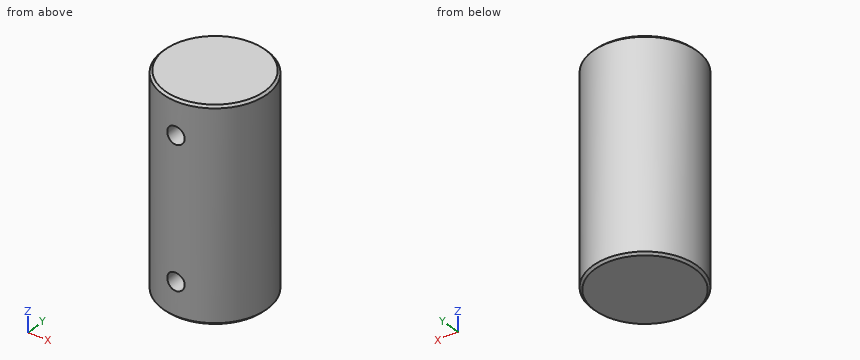
```python
from build123d import *

# Parameters (mm, degrees)
SKETCH1_R         = 9.525
EXTRUDE1_DEPTH    = 19.05
CHAMFER1_SIZE     = 0.4064
SKETCH6_R         = 1.5875
BLIND_HOLES_DEPTH = 7.62


with BuildPart() as part:
    # Sketch1 → Extrude1 (new body, symmetric)
    with BuildSketch(Plane.XY):
        Circle(SKETCH1_R)
    extrude(amount=EXTRUDE1_DEPTH, both=True)

    # Chamfer1
    chamfer1_edges = [part.edges().sort_by_distance(p)[0] for p in [
        (-9.525, 0, -19.05),
        (-9.525, 0, 19.05),
    ]]
    chamfer(chamfer1_edges, length=CHAMFER1_SIZE)

    # Sketch6 → Blind Holes (cut)
    with BuildSketch(Plane(origin=(0, -9.525, 0), x_dir=(-1, 0, 0), z_dir=(0, 1, 0))):
        with Locations(Location((0, 12.7, 0), (0, 0, 270))):  # turned: the seam where the file's is
            Circle(SKETCH6_R)
        with Locations(Location((0, -12.7, 0), (0, 0, 270))):  # turned: the seam where the file's is
            Circle(SKETCH6_R)
    extrude(amount=BLIND_HOLES_DEPTH, mode=Mode.SUBTRACT)


solid = part.part
```
Model file for the job. Use its own axes, mm. Give positions to 0.01 mm unless a question says otherwise; leave off trailing zeros. Loops run counter-clockwise (first coordinate to the right, second up) from the corner with the lowest first, then second, coordinate; pieces in that order, holes last. Notation, with made-up numbers: (58, 7.5) -> (66, 7.5) arc R22 cw to (66, 29.5) -> close; hole circle Ø10 at (32, 8). An arc over 180 degrees is marked (long way). Use CSV: the item, a comma, the result in double quotes. Start each with the question number.
1) Flat gauge pins, fed straight in: pin 1 Ø2 at (x, z) = (3, -5.5) entering from -Y; pin 2 Ø6 at (x, z) = (6, 5.5) entering from +Y; pin 3 Ø4 at (x, z) = (-6, 0.5) entering from -Y. Where does each tip first touch, or does it go through?
2) Slice it at C-C on y = -4.5. Give the number of separate pieces and of enclosed holes in the cut face, plus the area to 3 significant figures.
3) Slice it at B-B on z = 1.5. Give the cut face in (x, y) (3 decimals).
4) Wall check: line 1 (Y direction, x = 2.75, z = -13.5); line 2 (X direction, y = -6, z = -12.7); line 3 (X direction, y = -7.25, z = 12.7). Give the ranges that are in metal, low to high.
Computed values:
1,pin 1,"stops at y = -9.31"
1,pin 2,"stops at y = 9.04"
1,pin 3,"stops at y = -8.64"
2,separate pieces,"1"
2,enclosed holes,"2"
2,area,"623 mm^2"
3,outline,"circle Ø19.05 at (0, 0)"
4,line 1,"y = -9.12 to 9.12"
4,line 2,"x = -7.4 to -1.59, 1.59 to 7.4"
4,line 3,"x = -6.18 to -1.59, 1.59 to 6.18"
